Can you work these out from the model? Positions are in its coordinate system, mm. Face numbers are marked on the shaded views. A direction names the side the tool comes from. Give positions to 0.01 mm unless a question says otherwise; leave off trailing zeros. Order: outer loops, then holes, each group sorted by start corner. A loop starts at its lowest first (then second) coordinate and runs counter-clockwise, first axis right, second up. Notation, with made-up numbers: (-37, 73) - (15, 73) arc R8 cw to (15, 79) - close; hole circle Ø5 at (37.25, -9). An arc over 180 degrees is marked (long way). Return JSON: item names as keys, results as strings.
```python
from build123d import *

# Parameters (mm, degrees)
BOSS_EXTRUDE1_DEPTH = 7.5
SKETCH2_R           = 1.5
CUT_EXTRUDE1_DEPTH  = 9
CUT_EXTRUDE4_DEPTH  = 7
SKETCH6_R           = 1.25
BOSS_EXTRUDE2_DEPTH = 2
FILLET1_R           = 1
CUT_EXTRUDE5_DEPTH  = 3
SKETCH8_W           = 30
SKETCH8_H           = 7.5
CUT_EXTRUDE6_DEPTH  = 1.5


with BuildPart() as part:
    # Sketch1 → Boss-Extrude1 (new body)
    with BuildSketch(Plane(origin=(0, 0, 0), x_dir=(1, 0, 0), z_dir=(0, 1, 0))):
        with BuildLine():
            Line((0.6, -4.416738673), (-25.816064279, -4.416738673))
            ThreePointArc((-25.816064279, -4.416738673), (-27.230277841, -3.830952235), (-27.816064279, -2.416738673))
            Line((-27.816064279, -2.416738673), (-27.816064279, 1.242047676))
            ThreePointArc((-27.816064279, 1.242047676), (-27.230277841, 2.656261238), (-25.816064279, 3.242047676))
            Line((-25.816064279, 3.242047676), (-8.616701404, 3.242047676))
            ThreePointArc((-8.616701404, 3.242047676), (-6.877923642, 4.253790678), (-6.898342112, 6.265395781))
            Line((-6.898342112, 6.265395781), (-28.209840808, 42.050688808))
            ThreePointArc((-28.209840808, 42.050688808), (-29.932839186, 43.027335323), (-31.651288288, 42.042706201))
            Line((-31.651288288, 42.042706201), (-52.738515342, 6.257413174))
            ThreePointArc((-52.738515342, 6.257413174), (-52.751907933, 4.249760166), (-51.015427154, 3.242047676))
            Line((-51.015427154, 3.242047676), (-33.816064279, 3.242047676))
            ThreePointArc((-33.816064279, 3.242047676), (-32.401850716, 2.656261238), (-31.816064279, 1.242047676))
            Line((-31.816064279, 1.242047676), (-31.816064279, -2.416738673))
            ThreePointArc((-31.816064279, -2.416738673), (-32.401850716, -3.830952235), (-33.816064279, -4.416738673))
            Line((-33.816064279, -4.416738673), (-64.322377342, -4.416738673))
            ThreePointArc((-64.322377342, -4.416738673), (-66.058858122, -3.409026183), (-66.045465531, -1.401373175))
            Line((-66.045465531, -1.401373175), (-31.651288288, 56.965983893))
            ThreePointArc((-31.651288288, 56.965983893), (-29.932839186, 57.950613015), (-28.209840808, 56.973966501))
            Line((-28.209840808, 56.973966501), (4.418617661, 2.185752684))
            ThreePointArc((4.418617661, 2.185752684), (5.677744474, 1.262538298), (7.216741926, 1.52561999))
            Line((7.216741926, 1.52561999), (11.407599177, 4.21358701))
            ThreePointArc((11.407599177, 4.21358701), (12.276616363, 5.447347792), (12.036115602, 6.93715178))
            Line((12.036115602, 6.93715178), (7.323304576, 14.677687772))
            ThreePointArc((7.323304576, 14.677687772), (7.288002317, 16.697524788), (9.031585974, 17.717771743))
            Line((9.031585974, 17.717771743), (12.543887874, 17.717771743))
            ThreePointArc((12.543887874, 17.717771743), (13.523640919, 17.4613554), (14.252169272, 16.757855713))
            Line((14.252169272, 16.757855713), (25.293332405, -1.376654703))
            ThreePointArc((25.293332405, -1.376654703), (25.328634664, -3.396491718), (23.585051007, -4.416738673))
            Line((23.585051007, -4.416738673), (0.6, -4.416738673))
        make_face()
    extrude(amount=BOSS_EXTRUDE1_DEPTH)

    # Sketch2 → Cut-Extrude1 (cut)
    with BuildSketch(Plane(origin=(4.222678331, 0, -2.514765037), x_dir=(-0.5116740525225859, 0, -0.8591796459269238), z_dir=(0.8591796459269239, 0, -0.5116740525225859))):
        with Locations((57.281755723, 3.75)):
            Circle(SKETCH2_R)
    extrude(amount=-CUT_EXTRUDE1_DEPTH, mode=Mode.SUBTRACT)

    # Sketch5 → Cut-Extrude4 (cut)
    with BuildSketch(Plane(origin=(3.363498685, 0, -2.003090985), x_dir=(-0.5116740525225859, 0, -0.8591796459269238), z_dir=(0.8591796459269239, 0, -0.5116740525225859))):
        with BuildLine():
            ThreePointArc((59.687787147, 1.923672452), (60.293645506, 3.69481399), (59.625444471, 5.443388859))
            ThreePointArc((59.625444471, 5.443388859), (59.11581554, 5.480697337), (59.078507063, 4.971068407))
            ThreePointArc((59.078507063, 4.971068407), (59.57110599, 3.68201607), (59.124466188, 2.376327548))
            ThreePointArc((59.124466188, 2.376327548), (59.179799119, 1.868339521), (59.687787147, 1.923672452))
        make_face()
        with BuildLine():
            ThreePointArc((54.875724299, 1.923672452), (54.26986594, 3.69481399), (54.938066975, 5.443388859))
            ThreePointArc((54.938066975, 5.443388859), (55.447695906, 5.480697337), (55.485004384, 4.971068407))
            ThreePointArc((55.485004384, 4.971068407), (54.992405456, 3.68201607), (55.439045258, 2.376327548))
            ThreePointArc((55.439045258, 2.376327548), (55.383712327, 1.868339521), (54.875724299, 1.923672452))
        make_face()
    extrude(amount=-CUT_EXTRUDE4_DEPTH, mode=Mode.SUBTRACT)

    # Sketch6 → Boss-Extrude2 (add)
    with BuildSketch(Plane(origin=(11.862431053, 0, -7.222419211), x_dir=(0.5200419851467809, 0, 0.8541406989978848), z_dir=(-0.8541406989978848, 0, 0.5200419851467809))):
        with Locations(Location((-1.021383997, 3.75, 0), (0, 0, 180))):
            Circle(SKETCH6_R)
    extrude(amount=BOSS_EXTRUDE2_DEPTH)

    # Fillet1
    fillet1_edges = [part.edges().sort_by_distance(p)[0] for p in [
        (10.273039575, 3.75, -5.987065009),
    ]]
    fillet(fillet1_edges, radius=FILLET1_R)

    # Sketch7 → Cut-Extrude5 (cut)
    with BuildSketch(Plane.XZ.offset(-7.5)):
        Polygon((-17.79728073, -39.489672278), (-21.775246759, -37.120642694), (-16.658506234, -28.528846235), (-12.680540205, -30.897875819), align=None)
    extrude(amount=CUT_EXTRUDE5_DEPTH, mode=Mode.SUBTRACT)

    # Sketch8 → Cut-Extrude6 (cut)
    with BuildSketch(Plane(origin=(4.222678331, 0, -2.514765037), x_dir=(-0.5116740525225859, 0, -0.8591796459269238), z_dir=(0.8591796459269239, 0, -0.5116740525225859))):
        with Locations((32.718162055, 3.75)):
            Rectangle(SKETCH8_W, SKETCH8_H)
    extrude(amount=-CUT_EXTRUDE6_DEPTH, mode=Mode.SUBTRACT)


solid = part.part
```
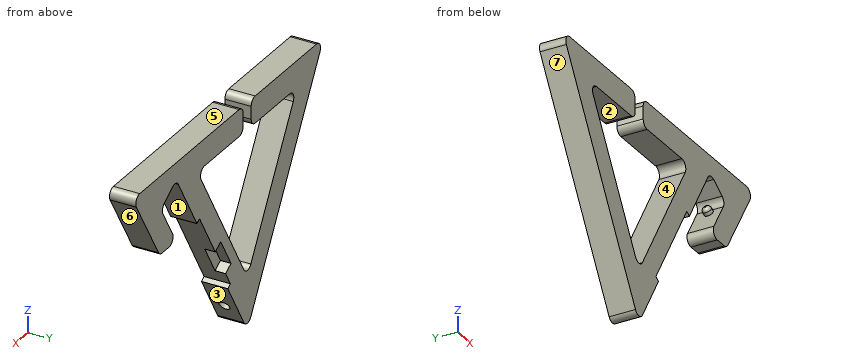
1. For pin 1 Ø1 at (y, z) = (1, -42) entering from +X; pin 2 Ø1.8 at (x, y) = (11.5, 3) entering from -Z; pin 3 Ø1.1 at (y, z) = (2, 1) entering from +X, each with a flat end and sliding along its axis, tell me the tip position at first contact or that it passes through.
Checks:
{"pin 1": "x = -20.74", "pin 2": "z = -17.72", "pin 3": "x = 25.39"}
2. Suppose I cut it at D-D (x = 16.5). List the corners of the cut face in (y, z) for me, plus the area to 3 significant figures.
Checks:
{"outline": "(0, -13.07) - (7.5, -13.07) - (7.5, 4.42) - (0, 4.42) - close", "area": "131 mm^2"}
3. On a 3-axis mill with a long thin cutter (end or side, diameter ignored), from which of +Z, -Z, +X, -X, +Y, -Y can I reach the whole of each face in a straight line? I mean the marked faces 1, 2 and 3. Say none if no direction works.
Checks:
{"face 1": "-Z, +Y, -Y", "face 2": "+Y, -Y", "face 3": "-Z, +X, +Y, -Y"}
4. Suppose I cut it at B-B (z = -19.5). List the corners of the cut face in (x, y) for me.
Checks:
{"outline": "(-53.73, 0) - (-44.94, 0) - (-44.94, 7.5) - (-53.73, 7.5) - close; (-14.78, 0) - (-7.64, 0) - (-7.64, 7.5) - (-14.78, 7.5) - close"}
5. If I drill on L1, parallel to Z at x = -30, y = 4.75; L2, parallel to X at y = 4.25, z = -10.5; L3, parallel to X at y = 4, z = -4, over which ranges is the centre line in solid material (lowest first)? Write a range as [from, to].
Checks:
{"L1": "[-57.95, -52.04], [-51.09, -50.11], [-47.5, -46.52], [-45.57, -43.03]", "L2": "[-59.03, -50.24], [-9.42, -0.53], [9.87, 18.06]", "L3": "[-62.86, -52.58], [-7.05, 3.34], [11.07, 22.02]"}
6. Thinking about a two-plate mould opening in X: for the marked faces 4, 5, 6 and 7, which applies, +X half, -X half, draft (parallel to the pull), parting line (faces both ways), or undercut?
Checks:
{"face 4": "undercut", "face 5": "draft", "face 6": "+X half", "face 7": "-X half"}
7. Suppose I cut it at C-C (z = -13). List the corners of the cut face in (x, y) for me.
Checks:
{"outline": "(-57.56, 0) - (-48.77, 0) - (-48.77, 7.5) - (-57.56, 7.5) - close; (-10.91, 0) - (-2.02, 0) - (-2.02, 7.5) - (-10.91, 7.5) - close; (8.34, 0) - (16.54, 0) - (16.54, 7.5) - (8.34, 7.5) - close"}
8. Suppose I cut it at A-A (x = -23). List the corners of the cut face in (y, z) for me, plus the area to 3 significant figures.
Checks:
{"outline": "(0, -48.23) - (7.5, -48.23) - (7.5, -33.3) - (0, -33.3) - close; (0, -3.24) - (7.5, -3.24) - (7.5, 4.42) - (0, 4.42) - close", "area": "169 mm^2"}
